Geometry: final body of the model. Coordinates: model frame, mm. A direction names the side the tool comes from. Give positions to 0.01 mm unless a question says otherwise; leave off trailing zeros. Write each loop counter-clockwise with the first axis right and the second up, starting at its lowest first coordinate (ties: lowest second). Pieces come first, ordered by that corner, then holes. Notation, with made-up numbers: M 43,69 L 99,69 A18 ccw 99,87 Z; hole C 7.5,76.5 d9. An arc over 180 degrees is marked long. Use one line per item in the form item = value. Start each with the question number.
Item 1: Section query D-D on x = 84. Give the number of separate pieces and of enclosed holes in the cut face, then the cut area to 3 significant figures.
Item 2: Section query A-A on z = 14. Return loops of the section in (x, y).
Item 3: Material intervals for line 1 along Z through (x, y) = (14.5, 5); line 2 along Z through (x, y) = (42, 0); line 3 along Z through (x, y) = (48.5, -13.5), sorted ascending. Write a range as from..to.
Item 4: Section query C-C on z = 0. Return loops of the section in (x, y).
Item 5: Contact query for a flat-ended pin moving along its axis: P1, Ø3, axis at x = 85, y = 6, coming from the +Z side. Output: stop coordinate, or through.
Item 6: Access query for faces 4 (the flat face through (51, -20, 10)), 5 (the flat face through (95, -4, 18)), 6 (the flat face through (51, -14, 18)). Directions: +Z, -Z, +X, -X, +Y, -Y. A direction counts if a zero-diameter tool reaches every point of the face in a straight line with its end or side. Return the directions, or none.
Item 7: Pull-direction query (Y, two-part tool) for faces 1 (the flat face through (51, 20, 10)), 2 (the flat face through (94, 0, 7.75)), 3 (the flat face through (51, -10, 20)); classes: released by +Y, released by -Y, zero draft, split by the parting line, or undercut.
Item 8: Section query B-B on y = 0. Return loops of the section in (x, z).
from build123d import *

# Parameters (mm, degrees)
SKIZZE11_R                     = 4
STRUKTURBAUTEIL1_DEPTH         = 100
SKIZZE2_R                      = 10
SCHNITT_LINEAR_AUSTRAGEN_DEPTH = 15.9


with BuildPart() as part:
    # Skizze11 → Strukturbauteil1 (new body)
    with BuildSketch(Plane(origin=(100, 0, 0), x_dir=(0, -1, 0), z_dir=(-1, 0, 0))):
        with BuildLine():
            Line((16, 20), (4, 20))
            Line((4, 20), (4, 15.5))
            Line((4, 15.5), (7, 15.5))
            Line((7, 15.5), (7, 18))
            Line((7, 18), (10, 18))
            Line((10, 18), (10, 12))
            Line((10, 12), (5.5, 7.75))
            Line((5.5, 7.75), (-5.5, 7.75))
            Line((-5.5, 7.75), (-10, 12))
            Line((-10, 12), (-10, 18))
            Line((-10, 18), (-7, 18))
            Line((-7, 18), (-7, 15.5))
            Line((-7, 15.5), (-4, 15.5))
            Line((-4, 15.5), (-4, 20))
            Line((-4, 20), (-16, 20))
            ThreePointArc((-16, 20), (-18.828427125, 18.828427125), (-20, 16))
            Line((-20, 16), (-20, 4))
            Line((-20, 4), (-15.5, 4))
            Line((-15.5, 4), (-15.5, 7))
            Line((-15.5, 7), (-18, 7))
            Line((-18, 7), (-18, 10))
            Line((-18, 10), (-12, 10))
            Line((-12, 10), (-7.75, 5.5))
            Line((-7.75, 5.5), (-7.75, -5.5))
            Line((-7.75, -5.5), (-12, -10))
            Line((-12, -10), (-18, -10))
            Line((-18, -10), (-18, -7))
            Line((-18, -7), (-15.5, -7))
            Line((-15.5, -7), (-15.5, -4))
            Line((-15.5, -4), (-20, -4))
            Line((-20, -4), (-20, -16))
            ThreePointArc((-20, -16), (-18.828427125, -18.828427125), (-16, -20))
            Line((-16, -20), (16, -20))
            ThreePointArc((16, -20), (18.828427125, -18.828427125), (20, -16))
            Line((20, -16), (20, -4))
            Line((20, -4), (15.5, -4))
            Line((15.5, -4), (15.5, -7))
            Line((15.5, -7), (18, -7))
            Line((18, -7), (18, -10))
            Line((18, -10), (12, -10))
            Line((12, -10), (7.75, -5.5))
            Line((7.75, -5.5), (7.75, 5.5))
            Line((7.75, 5.5), (12, 10))
            Line((12, 10), (18, 10))
            Line((18, 10), (18, 7))
            Line((18, 7), (15.5, 7))
            Line((15.5, 7), (15.5, 4))
            Line((15.5, 4), (20, 4))
            Line((20, 4), (20, 16))
            ThreePointArc((20, 16), (18.828427125, 18.828427125), (16, 20))
        make_face()
        Circle(SKIZZE11_R, mode=Mode.SUBTRACT)
        with BuildLine():
            Line((12, 18), (12, 12))
            Line((12, 12), (18, 12))
            Line((18, 12), (18, 16))
            ThreePointArc((18, 16), (17.414213562, 17.414213562), (16, 18))
            Line((16, 18), (12, 18))
        make_face(mode=Mode.SUBTRACT)
        with BuildLine():
            Line((-18, 12), (-12, 12))
            Line((-12, 12), (-12, 18))
            Line((-12, 18), (-16, 18))
            ThreePointArc((-16, 18), (-17.414213562, 17.414213562), (-18, 16))
            Line((-18, 16), (-18, 12))
        make_face(mode=Mode.SUBTRACT)
        Polygon((-4, -18), (4, -18), (4, -15.5), (7, -15.5), (7, -18), (10, -18), (10, -12), (5.5, -7.75), (-5.5, -7.75), (-10, -12), (-10, -18), (-7, -18), (-7, -15.5), (-4, -15.5), align=None, mode=Mode.SUBTRACT)
        with BuildLine():
            Line((18, -12), (12, -12))
            Line((12, -12), (12, -18))
            Line((12, -18), (16, -18))
            ThreePointArc((16, -18), (17.414213562, -17.414213562), (18, -16))
            Line((18, -16), (18, -12))
        make_face(mode=Mode.SUBTRACT)
        with BuildLine():
            Line((-12, -18), (-12, -12))
            Line((-12, -12), (-18, -12))
            Line((-18, -12), (-18, -16))
            ThreePointArc((-18, -16), (-17.414213562, -17.414213562), (-16, -18))
            Line((-16, -18), (-12, -18))
        make_face(mode=Mode.SUBTRACT)
    extrude(amount=STRUKTURBAUTEIL1_DEPTH)

    # Skizze2 → Schnitt-Linear austragen (cut)
    with BuildSketch(Plane(origin=(60.206991795, 21.446159487, 20), x_dir=(1, 0, 0), z_dir=(0, 0, 1))):
        with Locations(Location((19.793008205, -21.446159487, 0), (0, 0, 33.367012969))):  # turned: the seam where the file's is
            Circle(SKIZZE2_R)
    extrude(amount=-SCHNITT_LINEAR_AUSTRAGEN_DEPTH, mode=Mode.SUBTRACT)


solid = part.part
Answer sheet:
q1.separate_pieces = 3
q1.enclosed_holes = 6
q1.area = 555 mm2
q2.outline = M 0,-20 L 100,-20 L 100,-18 L 0,-18 Z; M 0,-12 L 100,-12 L 100,-10 L 0,-10 Z; M 0,10 L 100,10 L 100,12 L 0,12 Z; M 0,18 L 100,18 L 100,20 L 0,20 Z
q3.line_1 = -20..-15.5, -7.75..7.75, 15.5..20
q3.line_2 = -20..-18, -7.75..-4, 4..7.75
q3.line_3 = -20..-18, -12..-10, 10..12, 18..20
q4.outline = M 0,-7.75 L 100,-7.75 L 100,-4 L 0,-4 Z; M 0,4 L 100,4 L 100,7.75 L 0,7.75 Z
q5.P1 = 4.1
q6.face_4 = +Z, -Z, +X, -X, -Y
q6.face_5 = +Z, +X, -X
q6.face_6 = +X, -X
q7.face_1 = released by +Y
q7.face_2 = undercut
q7.face_3 = zero draft
q8.outline = M 0,-20 L 100,-20 L 100,-18 L 0,-18 Z; M 0,-7.75 L 100,-7.75 L 100,-4 L 0,-4 Z; M 0,4 L 100,4 L 100,7.75 L 90,7.75 L 90,4.1 L 70,4.1 L 70,7.75 L 0,7.75 Z
